Check sheet for the modelled part. Datum: model origin and axes. Units: mm. Coordinates: 2 decimals unless noted, no trailing zeros. Write each loop counter-clockwise with the first axis right and the second up, starting at its lowest first coordinate (ties: lowest second). Pieces come first, ordered by that corner, then holes. Notation, with made-up numbers: M -40,-10.75 L -30,-10.75 A17 ccw -30,1.25 Z; hole C 34.25,36 d8. An arc over 180 degrees is marked long. Answer as CSV lines item,"result". Start each with the question number.
Q1. Sectioned sample at A-A, the plane z = 15.5. Record the cut outline in (x, y).
Q2. Thickness scan on line 1 along Z through (x, y) = (-15.5, 1.35); line 2 along Z through (x, y) = (0, 1.05). Record the ranges inside material, lowest first. Write a range as from..to.
Q3. Sectioned sample at C-C, the plane x = -15.5. Record the cut outline in (y, z), then the cut area to 3 significant figures.
Q4. Mould release check, pull along X, two halves, no side actions. Record for faces 1 (the cylindrical face through (-17.07, 0.99, -14.85)), 2 (the flat face through (19.2, 1, 19.1)), 3 (the flat face through (9, 2, 9)): pulls with the +X half, pulls with the -X half, needs draft (parallel to the pull), parting line crosses it, or undercut.
Q5. Sectioned sample at B-B, the plane x = 0. Record the cut outline in (y, z).
Q6. Sectioned sample at D-D, the plane z = 0. Record the cut outline in (x, y).
from build123d import *

# Parameters (mm, degrees)
SKETCH1_W            = 42.3
SKETCH1_H            = 42.3
BOSS_EXTRUDE1_DEPTH  = 2
SKETCH2_R            = 11.25
CUT_EXTRUDE1_DEPTH   = 3
M3_CLEARANCE_HOLE1_D = 3.4
CHAMFER1_SIZE        = 4


with BuildPart() as part:
    # Sketch1 → Boss-Extrude1 (new body)
    with BuildSketch(Plane(origin=(0, 0, 0), x_dir=(1, 0, 0), z_dir=(0, 1, 0))):
        Rectangle(SKETCH1_W, SKETCH1_H)
    extrude(amount=BOSS_EXTRUDE1_DEPTH)

    # Sketch2 → Cut-Extrude1 (cut, through all)
    with BuildSketch(Plane(origin=(0, 2, 0), x_dir=(1, 0, 0), z_dir=(0, 1, 0))):
        Circle(SKETCH2_R)
    extrude(amount=-CUT_EXTRUDE1_DEPTH, mode=Mode.SUBTRACT)

    # M3 Clearance Hole1 (through all)
    with Locations(Plane(origin=(0, 2, 0), x_dir=(1, 0, 0), z_dir=(0, 1, 0))):
        with Locations((-15.5, 15.5), (15.5, 15.5), (15.5, -15.5), (-15.5, -15.5)):
            Hole(M3_CLEARANCE_HOLE1_D / 2)

    # Chamfer1
    chamfer1_edges = [part.edges().sort_by_distance(p)[0] for p in [
        (21.15, 1, 21.15),
        (-21.15, 1, 21.15),
        (-21.15, 1, -21.15),
        (21.15, 1, -21.15),
    ]]
    chamfer(chamfer1_edges, length=CHAMFER1_SIZE)


solid = part.part
Output:
1,outline,"M -21.15,0 L -17.2,0 L -17.2,2 L -21.15,2 Z; M -13.8,0 L 13.8,0 L 13.8,2 L -13.8,2 Z; M 17.2,0 L 21.15,0 L 21.15,2 L 17.2,2 Z"
2,line 1,"z = -21.15..-17.2, -13.8..13.8, 17.2..21.15"
2,line 2,"z = -21.15..-11.25, 11.25..21.15"
3,outline,"M 0,-21.15 L 2,-21.15 L 2,-17.2 L 0,-17.2 Z; M 0,-13.8 L 2,-13.8 L 2,13.8 L 0,13.8 Z; M 0,17.2 L 2,17.2 L 2,21.15 L 0,21.15 Z"
3,area,"71.0 mm^2"
4,face 1,"undercut"
4,face 2,"pulls with the +X half"
4,face 3,"needs draft"
5,outline,"M 0,-21.15 L 2,-21.15 L 2,-11.25 L 0,-11.25 Z; M 0,11.25 L 2,11.25 L 2,21.15 L 0,21.15 Z"
6,outline,"M -21.15,0 L -11.25,0 L -11.25,2 L -21.15,2 Z; M 11.25,0 L 21.15,0 L 21.15,2 L 11.25,2 Z"
